The model under review builds one solid part; all positions refer to its coordinate system, in mm. Face numbers are marked on the shaded views. A direction names the side the tool comes from. Coordinates: 2 decimals unless noted, no trailing zeros. Loops run counter-clockwise (first coordinate to the right, second up) from the corner with the lowest first, then second, coordinate; pieces in that order, holes last. Notation, with made-up numbers: (-40, -12) - (-15, -12) arc R7 cw to (-15, -4) - close; hole circle Ø5 at (89.25, 38). An arc over 180 degrees is marked (long way). One line per item, written item: value. Start each with the question number.
1. We need section D-D, the plane x = -23. Count the separate pieces of the cut face and the enclosed holes in it, then the cut area to 3 significant figures.
2. Insertion check: P1, Ø6.5, axis at x = -23, y = 21, coming from the -Z side; P2, Ø12, axis at x = -23.5, y = 19, coming from the -Z side; P3, Ø1, axis at x = -18, z = 11, coming from the +Y side; P4, Ø5, axis at x = 23, y = 8, coming from the -Z side. Each pin has a flat end and moves straight along its axis. Give the tip position at first contact, or say it passes through.
3. Mouldability with a two-part tool opening along X and no side actions: class the marked faces 1, 2, 3 and 4 as +X half, -X half, draft (parallel to the pull), parting line (faces both ways), or undercut.
4. To check wall thickness, follow line 1 (Z direction, x = 11, y = 31.9); line 2 (X direction, y = 32.1, z = -19.75); line 3 (Z direction, x = 23, y = 26). State the ranges of each line that lie inside material, in increasing order.
5. We need section A-A, the plane x = 0. Give the boundary of the cut face in (y, z), then the cut area to 3 significant figures.
6. We need section C-C, the plane x = -11. Give the boundary of the cut face in (y, z).
7. We need section B-B, the plane z = 13. Give the boundary of the cut face in (x, y), then the cut area to 3 significant figures.
8. For the marked faces 5, 6 and 7, list the 3-axis set-ups (+Z, -Z, +X, -X, +Y, -Y) from which the entire face can be reached by the end or side of a thin tool; tool diameter is ignored.
from build123d import *

# Parameters (mm, degrees)
SKETCH_1_W                  = 60
SKETCH_1_H                  = 32.5
SKETCH_1_R                  = 6
SKETCH_1_R_2                = 2.75
EXTRUDE_1_DEPTH             = 29
SKETCH_2_W                  = 34
SKETCH_2_H                  = 34
SKETCH_2_R                  = 6
EXTRUDE_2_DEPTH             = 34
SKETCH_3_R                  = 3
CUT_EXTRUDE_1_DEPTH         = 3
CHAMFER_1_SIZE              = 2
FILLET_1_R                  = 1
HOLE_WIZARD_M5_1_AT_2_COUNT = 2
HOLE_WIZARD_M5_1_AT_2_PITCH = 13
HOLE_WIZARD_M5_1_AT_3_COUNT = 2
HOLE_WIZARD_M5_1_AT_3_PITCH = 46
HOLE_WIZARD_M5_1_AT_4_COUNT = 2
HOLE_WIZARD_M5_1_AT_4_PITCH = 47.801673611


with BuildPart() as part:
    # 草图1 → 凸台-拉伸1 (new body)
    with BuildSketch(Plane(origin=(0, 0, 0), x_dir=(1, 0, 0), z_dir=(0, 1, 0))):
        Rectangle(SKETCH_1_W, SKETCH_1_H)
        with Locations((0, 8.75)):
            Circle(SKETCH_1_R, mode=Mode.SUBTRACT)
        with Locations((-23, 8.75)):
            Circle(SKETCH_1_R_2, mode=Mode.SUBTRACT)
        with Locations((-23, -9.25)):
            Circle(SKETCH_1_R_2, mode=Mode.SUBTRACT)
        with Locations((23, -9.25)):
            Circle(SKETCH_1_R_2, mode=Mode.SUBTRACT)
        with Locations((23, 8.75)):
            Circle(SKETCH_1_R_2, mode=Mode.SUBTRACT)
    extrude(amount=EXTRUDE_1_DEPTH)

    # 草图2 → 凸台-拉伸2 (add)
    with BuildSketch(Plane.XZ):
        with Locations((0, -8.75)):
            Rectangle(SKETCH_2_W, SKETCH_2_H)
        with Locations((0, -8.75)):
            Circle(SKETCH_2_R, mode=Mode.SUBTRACT)
    extrude(amount=-EXTRUDE_2_DEPTH)

    # 草图3 → 切除-拉伸1 (cut)
    with BuildSketch(Plane(origin=(0, 34, 0), x_dir=(1, 0, 0), z_dir=(0, 1, 0))):
        with Locations((-11, 19.75)):
            Circle(SKETCH_3_R)
        with Locations((11, 19.75)):
            Circle(SKETCH_3_R)
        with Locations((-11, -2.25)):
            Circle(SKETCH_3_R)
        with Locations((11, -2.25)):
            Circle(SKETCH_3_R)
    extrude(amount=-CUT_EXTRUDE_1_DEPTH, mode=Mode.SUBTRACT)

    # 倒角1
    chamfer_1_edges = [part.edges().sort_by_distance(p)[0] for p in [
        (-17, 17, -25.75),
        (17, 17, -25.75),
        (30, 14.5, 16.25),
        (-30, 14.5, 16.25),
    ]]
    chamfer(chamfer_1_edges, length=CHAMFER_1_SIZE)

    # 圆角1
    fillet_1_edges = [part.edges().sort_by_distance(p)[0] for p in [
        (-30, 29, -1),
        (-17, 0, -20),
        (-17, 29, -4),
        (-17, 34, -7.75),
        (17, 29, -4),
        (-30, 0, -1),
        (17, 0, -20),
        (30, 0, -1),
        (30, 29, -1),
        (17, 34, -7.75),
    ]]
    fillet(fillet_1_edges, radius=FILLET_1_R)

    # 草图7 → M5 六角头螺栓的柱形沉头孔1 (revolve, cut)
    with BuildSketch(Plane(origin=(-23, 8, -16.25), x_dir=(0, 1, 0), z_dir=(1, 0, 0))):
        Polygon((0, 0), (0, 32.5), (2.75, 32.5), (2.75, 0.5), (5.5, 0.5), (5.5, 0.025), (5.525, 0), align=None)
    hole_wizard_m5_1 = revolve(axis=Axis((-23, 8, -22.6), (0, 0, 1)), mode=Mode.SUBTRACT)

    # M5 六角头螺栓的柱形沉头孔1 at 2: M5 六角头螺栓的柱形沉头孔1 ×2
    with Locations(*[(0, i * HOLE_WIZARD_M5_1_AT_2_PITCH, 0) for i in range(1, HOLE_WIZARD_M5_1_AT_2_COUNT)]):
        add(hole_wizard_m5_1, mode=Mode.SUBTRACT)

    # M5 六角头螺栓的柱形沉头孔1 at 3: M5 六角头螺栓的柱形沉头孔1 ×2
    with Locations(*[(i * HOLE_WIZARD_M5_1_AT_3_PITCH, 0, 0) for i in range(1, HOLE_WIZARD_M5_1_AT_3_COUNT)]):
        add(hole_wizard_m5_1, mode=Mode.SUBTRACT)

    # M5 六角头螺栓的柱形沉头孔1 at 4: M5 六角头螺栓的柱形沉头孔1 ×2
    with Locations(*[Vector(0.962309403, 0.271957005, 0) * (i * HOLE_WIZARD_M5_1_AT_4_PITCH) for i in range(1, HOLE_WIZARD_M5_1_AT_4_COUNT)]):
        add(hole_wizard_m5_1, mode=Mode.SUBTRACT)


solid = part.part
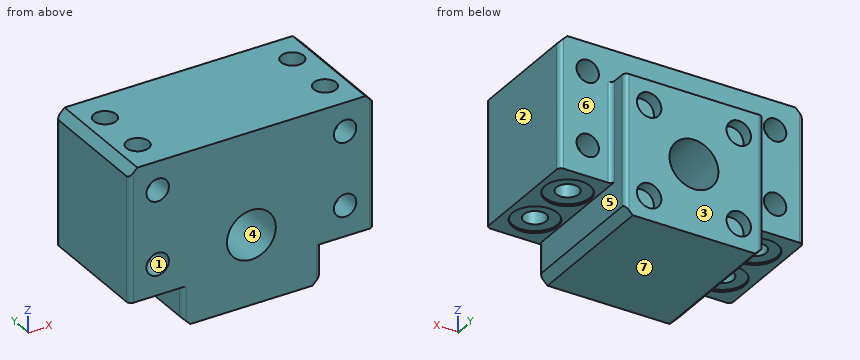
Findings below:
1. separate pieces: 9
1. enclosed holes: 0
1. area: 381 mm2
2. P1: z = -15.75
2. P2: z = -16.25
2. P3: y = 29
2. P4: through
3. face 1: undercut
3. face 2: +X half
3. face 3: draft
3. face 4: undercut
4. line 1: -25.75 to -22.75, -16.75 to -0.75, 5.25 to 8.25
4. line 2: -17 to -14, -8 to 8, 14 to 17
4. line 3: -15.75 to -11.5, -6 to 6.5, 12 to 16.25
5. outline: (0, -25.75) - (34, -25.75) - (34, -14.75) - (0, -14.75) - close; (0, -2.75) - (34, -2.75) - (34, 8.25) - (29, 8.25) - (29, 16.25) - (0, 16.25) - close
5. area: 980 mm2
6. outline: (0, -25.75) - (34, -25.75) - (34, -22.75) - (31, -22.75) - (31, -16.75) - (34, -16.75) - (34, -0.75) - (31, -0.75) - (31, 5.25) - (34, 5.25) - (34, 8.25) - (29, 8.25) - (29, 16.25) - (0, 16.25) - close
7. outline: (-30, 1) arc R1 ccw to (-29, 0) - (29, 0) arc R1 ccw to (30, 1) - (30, 28) arc R1 ccw to (29, 29) - (-29, 29) arc R1 ccw to (-30, 28) - close; hole circle Ø5.5 at (-23, 8); hole circle Ø5.5 at (-23, 21); hole circle Ø5.5 at (23, 8); hole circle Ø5.5 at (23, 21)
7. area: 1,640 mm2
8. face 5: -Z, +X, +Y
8. face 6: +Z, +Y
8. face 7: -Z, +X, -X, +Y, -Y
